```python
from build123d import *

# Parameters (mm, degrees)
ESQUISSE1_R                  = 25
BOSS_EXTRU_1_DEPTH           = 4
ENL_V_MAT_EXTRU_1_DEPTH      = 107.066017178
ENL_V_MAT_EXTRU_1_DEPTH_BACK = 107.066017178
ESQUISSE2_R                  = 4.5


with BuildPart() as part:
    # Esquisse1 → Boss.-Extru.1 (new body)
    with BuildSketch(Plane(origin=(0, 0, 0), x_dir=(1, 0, 0), z_dir=(0, 1, 0))):
        with Locations(Location((0, 0, 0), (0, 0, 270))):
            Circle(ESQUISSE1_R)
    extrude(amount=BOSS_EXTRU_1_DEPTH)

    # Esquisse3 → R_volution1 (revolve)
    with BuildSketch(Plane(origin=(0, 0, 0), x_dir=(0, 0, -1), z_dir=(1, 0, 0))):
        Polygon((0, 4), (-16, 4), (-13, 104), (0, 104), align=None)
    revolve(axis=Axis((0, 104, 0), (0, -1, 0)))

    # Esquisse2 → Enl_v. mat.-Extru.1 (cut, two sides: drawn at the far end of the back side and taken through both)
    with BuildSketch(Plane(origin=(0, 4, 0), x_dir=(1, 0, 0), z_dir=(0, 1, 0)).offset(-ENL_V_MAT_EXTRU_1_DEPTH_BACK)):
        with Locations(Location((0, 0, 0), (0, 0, 270))):
            Circle(ESQUISSE2_R)
    extrude(amount=ENL_V_MAT_EXTRU_1_DEPTH + ENL_V_MAT_EXTRU_1_DEPTH_BACK, mode=Mode.SUBTRACT)


solid = part.part
```
Verification items for the finished model (mm, model axes). Give positions to 0.01 mm unless a question says otherwise; leave off trailing zeros. Order: outer loops, then holes, each group sorted by start corner. A loop starts at its lowest first (then second) coordinate and runs counter-clockwise, first axis right, second up. Notation, with made-up numbers: (33, 75) -> (54, 75) arc R7 ccw to (54, 83) -> close; hole circle Ø4 at (3.5, 1). An arc over 180 degrees is marked (long way). Use a Markdown table: item, result.
1) Material ranges on probe 1 along Y at (x, z) = (-11.5, -18.5); probe 2 along Z at (x, y) = (0, 23.5) (3 decimals); probe 3 along Z at (x, y) = (0, 64), recorded low to high.
Results:
| item | result |
|---|---|
| probe 1 | 0 to 4 |
| probe 2 | -15.415 to -4.5, 4.5 to 15.415 |
| probe 3 | -14.2 to -4.5, 4.5 to 14.2 |
2) Mould release check, pull along X, two halves, no side actions. Record for faces 1 (the conical face through (12.845, 54.7, 6.681)), 2 (the cylindrical face through (1.352, 51.272, 4.292)), 3 (the flat face through (-16.3, 4, -0.4)): pulls with the +X half, pulls with the -X half, needs draft (parallel to the pull), parting line crosses it, or undercut.
Results:
| item | result |
|---|---|
| face 1 | parting line crosses it |
| face 2 | undercut |
| face 3 | needs draft |
3) Depth check by flat-ended pin: pin 1 Ø12 at (y, z) = (69.5, -14) entering from +X; pin 2 Ø1.5 at (x, y) = (-12, 78) entering from +Z; pin 3 Ø3 at (x, y) = (6, 68.5) entering from +Z; pin 4 Ø12 at (x, z) = (-3, 17) entering from +Y. Enter the tip coordinate at first touch or a pass-through.
Results:
| item | result |
|---|---|
| pin 1 | x = 11.54 |
| pin 2 | z = 7.96 |
| pin 3 | z = 13.33 |
| pin 4 | y = 104 |
4) Section check B-B, the plane x = 0. Record the boundary of the cut face in (y, z).
Results:
| item | result |
|---|---|
| outline | (0, -25) -> (4, -25) -> (4, -16) -> (104, -13) -> (104, -4.5) -> (0, -4.5) -> close; (0, 4.5) -> (104, 4.5) -> (104, 13) -> (4, 16) -> (4, 25) -> (0, 25) -> close |
5) Section check D-D, the plane y = 56. Record the boundary of the cut face in (x, z), then the cut area to 3 significant figures.
Results:
| item | result |
|---|---|
| outline | circle Ø28.88 at (0, 0); hole circle Ø9 at (0, 0) |
| area | 591 mm² |
6) Section check A-A, the plane z = 0. Record the boundary of the cut face in (x, y), then the cut area to 3 significant figures.
Results:
| item | result |
|---|---|
| outline | (-25, 0) -> (-4.5, 0) -> (-4.5, 104) -> (-13, 104) -> (-16, 4) -> (-25, 4) -> close; (4.5, 0) -> (25, 0) -> (25, 4) -> (16, 4) -> (13, 104) -> (4.5, 104) -> close |
| area | 2,160 mm² |
7) Section check C-C, the plane y = 29. Record the boundary of the cut face in (x, z), then the cut area to 3 significant figures.
Results:
| item | result |
|---|---|
| outline | circle Ø30.5 at (0, 0); hole circle Ø9 at (0, 0) |
| area | 667 mm² |
